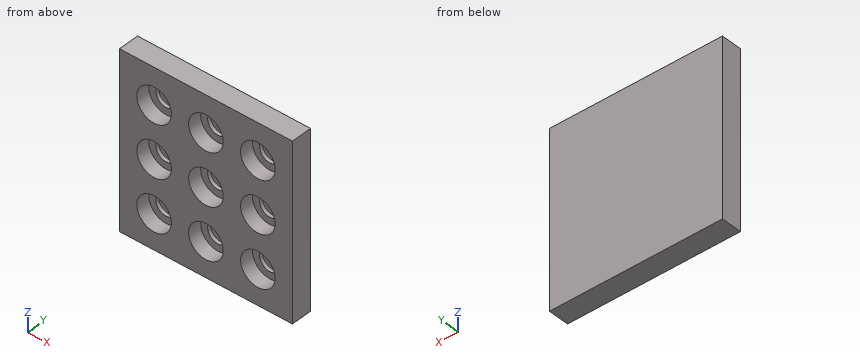
```python
from build123d import *

# Parameters (mm, degrees)
SKETCH_1_W                  = 25
SKETCH_1_H                  = 25.22650516
EXTRUDE_1_DEPTH             = 3
SKETCH_1_3_R                = 2.5
CUT_EXTRUDE_1_DEPTH         = 2
PATTERN_LINEAR_1_COUNT      = 3
PATTERN_LINEAR_1_PITCH      = 7.5
PATTERN_LINEAR_1_COUNT_DIR2 = 3
PATTERN_LINEAR_1_PITCH_DIR2 = 7.5
SKETCH_1_4_R                = 1.5
CUT_EXTRUDE_2_DEPTH         = 2.5
PATTERN_LINEAR_2_COUNT      = 3
PATTERN_LINEAR_2_PITCH      = 7.5
PATTERN_LINEAR_2_COUNT_DIR2 = 3
PATTERN_LINEAR_2_PITCH_DIR2 = 7.5


with BuildPart() as part:
    # Sketch 1 → Extrude 1 (new body)
    with BuildSketch(Plane(origin=(0, 0, 0), x_dir=(1, 0, 0), z_dir=(0, 1, 0))):
        with Locations((7.5, -7.38674742)):
            Rectangle(SKETCH_1_W, SKETCH_1_H)
    extrude(amount=EXTRUDE_1_DEPTH)

    # Sketch 1_3 → Cut-Extrude 1 (cut)
    with BuildSketch(Plane(origin=(0, 0, 0), x_dir=(1, 0, 0), z_dir=(0, 1, 0))):
        with Locations(Location((15, -14.77349484, 0), (0, 0, 270))):
            Circle(SKETCH_1_3_R)
    cut_extrude_1 = extrude(amount=CUT_EXTRUDE_1_DEPTH, mode=Mode.SUBTRACT)

    # Pattern Linear 1: Cut-Extrude 1 3 × 3
    with Locations(*[(-j * PATTERN_LINEAR_1_PITCH_DIR2, 0, -i * PATTERN_LINEAR_1_PITCH) for i in range(PATTERN_LINEAR_1_COUNT) for j in range(PATTERN_LINEAR_1_COUNT_DIR2) if (i, j) != (0, 0)]):
        add(cut_extrude_1, mode=Mode.SUBTRACT)

    # Sketch 1_4 → Cut-Extrude 2 (cut)
    with BuildSketch(Plane(origin=(0, 0, 0), x_dir=(1, 0, 0), z_dir=(0, 1, 0))):
        with Locations(Location((15, -14.77349484, 0), (0, 0, 270))):
            Circle(SKETCH_1_4_R)
    cut_extrude_2 = extrude(amount=CUT_EXTRUDE_2_DEPTH, mode=Mode.SUBTRACT)

    # Pattern Linear 2: Cut-Extrude 2 3 × 3
    with Locations(*[(-j * PATTERN_LINEAR_2_PITCH_DIR2, 0, -i * PATTERN_LINEAR_2_PITCH) for i in range(PATTERN_LINEAR_2_COUNT) for j in range(PATTERN_LINEAR_2_COUNT_DIR2) if (i, j) != (0, 0)]):
        add(cut_extrude_2, mode=Mode.SUBTRACT)


solid = part.part
```
CAD build for the part. Positions are in the model's coordinates, mm. Give positions to 0.01 mm unless a question says otherwise; leave off trailing zeros. Loops run counter-clockwise (first coordinate to the right, second up) from the corner with the lowest first, then second, coordinate; pieces in that order, holes last. Notation, with made-up numbers: (64, -2.5) - (91, -2.5) arc R15 ccw to (91, 19.5) - close; hole circle Ø3 at (89.5, 10). An arc over 180 degrees is marked (long way). Put each result on its own line as item: value.
Q1. Slice it at A-A (y = 1.55). Give the number of separate pieces and of enclosed holes in the cut face, plus the area to 3 significant figures.
Filled in:
separate pieces: 1
enclosed holes: 9
area: 454 mm²
Q2. Probe line 1 along Z through (x, y) = (0, 2.2); line 2 along X through (y, z) = (0.35, -0.25); line 3 along X through (y, z) = (1.9, 6). List the from-to ranges inside material, lowest first.
Filled in:
line 1: z = -5.23 to -1.73, 1.27 to 5.77, 8.77 to 13.27, 16.27 to 20
line 2: x = -5 to -2.5, 2.5 to 5, 10 to 12.5, 17.5 to 20
line 3: x = -5 to -2.15, 2.15 to 5.35, 9.65 to 12.85, 17.15 to 20
Q3. Slice it at B-B (x = 15). Give the cut face in (y, z).
Filled in:
outline: (0, -5.23) - (3, -5.23) - (3, 20) - (0, 20) - (0, 17.27) - (2, 17.27) - (2, 16.27) - (2.5, 16.27) - (2.5, 13.27) - (2, 13.27) - (2, 12.27) - (0, 12.27) - (0, 9.77) - (2, 9.77) - (2, 8.77) - (2.5, 8.77) - (2.5, 5.77) - (2, 5.77) - (2, 4.77) - (0, 4.77) - (0, 2.27) - (2, 2.27) - (2, 1.27) - (2.5, 1.27) - (2.5, -1.73) - (2, -1.73) - (2, -2.73) - (0, -2.73) - close
Q4. Slice it at C-C (z = 0). Give the cut face in (x, y).
Filled in:
outline: (-5, 0) - (-2.49, 0) - (-2.49, 2) - (-1.48, 2) - (-1.48, 2.5) - (1.48, 2.5) - (1.48, 2) - (2.49, 2) - (2.49, 0) - (5.01, 0) - (5.01, 2) - (6.02, 2) - (6.02, 2.5) - (8.98, 2.5) - (8.98, 2) - (9.99, 2) - (9.99, 0) - (12.51, 0) - (12.51, 2) - (13.52, 2) - (13.52, 2.5) - (16.48, 2.5) - (16.48, 2) - (17.49, 2) - (17.49, 0) - (20, 0) - (20, 3) - (-5, 3) - close
Q5. Flat gauge pins, fed straight in: pin 1 (3 mm diameter, centred on x = 15, z = 0.5, fed in from -Y); pin 2 (6 mm diameter, centred on x = 0, z = 7.27, fed in from -Y); pin 3 (0.9 mm diameter, centred on x = 0, z = 7.5, fed in from -Y). Where does each tip first touch, or does it go through?
Filled in:
pin 1: stops at y = 2
pin 2: stops at y = 0
pin 3: stops at y = 2.5
